from build123d import *

# Parameters (mm, degrees)
F0_W     = 20
F0_H     = 10
F0_W_2   = 10
F0_H_2   = 20
F1_DEPTH = 1.2


with BuildPart() as f1:
    # F0 (on Top) → F1 (new body)
    with BuildSketch(Plane.XY):
        with Locations((-15, 0)):
            Rectangle(F0_W, F0_H)
        Polygon((-23.952800427, 2.2430510182), (-23.6059203744, 2.5555547327), (-22.9180995375, 3.1808458734), (-21.4581449046, 1.5748944182), (-20.0015842271, 2.899039368), (-19.379123235, 2.2143316973), (-20.7127477867, 1.0019467672), (-19.4734830842, -0.3612455592), (-20.4429661396, -1.2425930456), (-21.572595225, 0), (-23.0182641957, -1.3142434066), (-23.7418717627, -0.5182744093), (-22.4829424203, 0.6262058426), align=None, mode=Mode.SUBTRACT)
        Rectangle(F0_W_2, F0_H)
        with Locations((15, 0)):
            Rectangle(F0_W, F0_H)
        with Locations((0, 15)):
            Rectangle(F0_W_2, F0_H_2)
        with Locations((0, -15)):
            Rectangle(F0_W_2, F0_H_2)
        Polygon((-0.4832326085, -19.6910500526), (-2.4245390669, -17.8273953497), (-1.6327861698, -16.4912146452), (0.8914793769, -18.8802530514), (2.5726677996, -17.1039040391), (3.0499449931, -17.5556130707), (0.9921601741, -19.7298750281), (0.9921601741, -23.1077484787), (-0.4832326085, -23.1077484787), align=None, mode=Mode.SUBTRACT)
    extrude(amount=F1_DEPTH)


solid = f1.part
Here's how the part is built. I have some questions about the finished solid (model axes, mm). A direction names the side the tool comes from. Give positions to 0.01 mm unless a question says otherwise; leave off trailing zeros. Loops run counter-clockwise (first coordinate to the right, second up) from the corner with the lowest first, then second, coordinate; pieces in that order, holes last. Notation, with made-up numbers: (4, -12) -> (52, -12) arc R29 ccw to (52, 20) -> close; hole circle Ø1 at (77, 88.25). An arc over 180 degrees is marked (long way). Answer as a JSON object with one key per item and string values. Group by question number.
Item 1: I need wall thicknesses on L1, parallel to X at y = -17.5, z = 0.5; L2, parallel to X at y = 5.5, z = 0.85; L3, parallel to X at y = -19, z = 1.15. Which ranges of each line are inside material? Lowest first, please.
Item 2: On a 3-axis mill with a long thin cutter (end or side, diameter ignored), from which of +Z, -Z, +X, -X, +Y, -Y can I reach the whole of each face in a straight line? I mean faces 4 (the flat face through (-15, 5, 1)), 5 (the flat face through (-5, -15, 1)), 6 (the flat face through (-20.74, 2.23, 0.59)). Say none if no direction works.
Item 3: Imagine slicing it at B-B on x = 19.5. Write out the boundary of the cut face in (y, z).
Item 4: Imagine slicing it at A-A on z = 0.2. Give the number of separate pieces and of enclosed holes in the cut face, then the cut area to 3 significant figures.
Item 5: Thinking about a two-plate mould opening in Y: for faces 1 (the flat face through (-0.483, -21, 1)), 2 (the flat face through (5, -15, 1)), 3 (the flat face through (0, 25, 1)), which applies, pulls with the +Y half, pulls with the -Y half, needs draft (parallel to the pull), parting line crosses it, or undercut?
Item 6: Will these pins go through, and if not, where does the flat tip stop? pin 1 (0.6 mm diameter, centred on y = 15, z = 0.5, fed in from -X); pin 2 (10 mm diameter, centred on x = -12.5, y = -7, fed in from -Z).
Answer list:
{
 "1": {"L1": "x = -5 to -2.23, -0.57 to 2.2, 2.99 to 5", "L2": "x = -5 to 5", "L3": "x = -5 to -1.2, 1.68 to 5"},
 "2": {"face 4": "+Z, -Z, -X, +Y", "face 5": "+Z, -Z, -X, -Y", "face 6": "+Z, -Z"},
 "3": {"outline": "(-5, 0) -> (5, 0) -> (5, 1.2) -> (-5, 1.2) -> close"},
 "4": {"separate pieces": "1", "enclosed holes": "2", "area": "877 mm2"},
 "5": {"face 1": "undercut", "face 2": "needs draft", "face 3": "pulls with the +Y half"},
 "6": {"pin 1": "stops at x = -5", "pin 2": "stops at z = 0"}
}
